Part model, mm, in its own coordinate system. Coordinates: 2 decimals unless noted, no trailing zeros. Loops run counter-clockwise (first coordinate to the right, second up) from the corner with the lowest first, then second, coordinate; pieces in that order, holes last. Notation, with made-up numbers: (34, -36) - (43, -36) arc R23 ccw to (43, -2) - close; hole circle Ø5 at (41.5, 83.25). An arc over 180 degrees is marked (long way). Use a Markdown table: item, result. Add a question column.
1) Band-saw the part on C-C (z = 10.5). Give the cut face in (x, y), plus the area to 3 significant figures.
2) Drop a flat-ended pin along its axis: P1, Ø3, axis at x = -77.4, z = 43.9, coming from the -Y side. Give the stop position or say it passes through.
3) Probe probe 1 along X at (y, z) = (2.9, -40); probe 2 along Z at (x, y) = (8, 3.5); probe 3 along X at (y, z) = (0.45, 41). List the from-to ranges inside material, lowest first. Write a range as [from, to].
4) Band-saw the part on D-D (y = 2.9). Give the number of separate pieces and of enclosed holes in the cut face, plus the area to 3 significant figures.
5) Band-saw the part on A-A (z = 40). Give the cut face in (x, y), plus the area to 3 significant figures.
6) Band-saw the part on B-B (x = -77.4). Give the cut face in (y, z).
from build123d import *

# Parameters (mm, degrees)
SKETCH1_W               = 161
SKETCH1_H               = 100
BOSS_EXTRUDE1_DEPTH     = 4
SKETCH2_R               = 1.75
CUT_EXTRUDE1_DEPTH      = 95.84856351
MIRROR2_COPY_1_SKETCH_R = 1.75
MIRROR2_COPY_1_DEPTH    = 95.84856351
SKETCH3_W               = 15
SKETCH3_H               = 60
CUT_EXTRUDE2_DEPTH      = 95.84856351
SKETCH4_R               = 1.6
CUT_EXTRUDE3_DEPTH      = 95.84856351
MIRROR5_COPY_1_SKETCH_R = 1.6
MIRROR5_COPY_1_DEPTH    = 95.84856351
SKETCH5_R               = 2.1
CUT_EXTRUDE4_DEPTH      = 95.84856351
SKETCH6_W               = 10
SKETCH6_H               = 40
CUT_EXTRUDE5_DEPTH      = 95.84856351
FILLET1_R               = 5


with BuildPart() as part:
    # Sketch1 → Boss-Extrude1 (new body)
    with BuildSketch(Plane(origin=(0, 0, 0), x_dir=(1, 0, 0), z_dir=(0, 1, 0))):
        Rectangle(SKETCH1_W, SKETCH1_H)
    extrude(amount=BOSS_EXTRUDE1_DEPTH)

    # Sketch2 → Cut-Extrude1 (cut, through all)
    with BuildSketch(Plane(origin=(0, 4, 0), x_dir=(1, 0, 0), z_dir=(0, 1, 0))):
        with Locations(Location((77.4, -43.9, 0), (0, 0, 270))):
            Circle(SKETCH2_R)
    cut_extrude1 = extrude(amount=-CUT_EXTRUDE1_DEPTH, mode=Mode.SUBTRACT)

    # Mirror1: Cut-Extrude1 across plane
    add(cut_extrude1.mirror(Plane.XY), mode=Mode.SUBTRACT)

    # Mirror2: Cut-Extrude1 across plane
    add(cut_extrude1.mirror(Plane(origin=(0, 0, 0), x_dir=(0, 0, 1), z_dir=(1, 0, 0))), mode=Mode.SUBTRACT)

    # Mirror2 copy 1 sketch → Mirror2 copy 1 (cut, through all)
    with BuildSketch(Plane(origin=(0, 4, 0), x_dir=(-1, 0, 0), z_dir=(0, 1, 0))):
        with Locations(Location((77.4, -43.9, 0), (0, 0, 270))):
            Circle(MIRROR2_COPY_1_SKETCH_R)
    extrude(amount=-MIRROR2_COPY_1_DEPTH, mode=Mode.SUBTRACT)

    # Sketch3 → Cut-Extrude2 (cut, through all)
    with BuildSketch(Plane(origin=(0, 4, 0), x_dir=(1, 0, 0), z_dir=(0, 1, 0))):
        with Locations((-27.5, -20)):
            Rectangle(SKETCH3_W, SKETCH3_H)
    cut_extrude2 = extrude(amount=-CUT_EXTRUDE2_DEPTH, mode=Mode.SUBTRACT)

    # Mirror3: Cut-Extrude2 across plane
    add(cut_extrude2.mirror(Plane(origin=(0, 0, 0), x_dir=(0, 0, 1), z_dir=(1, 0, 0))), mode=Mode.SUBTRACT)

    # Sketch4 → Cut-Extrude3 (cut, through all)
    with BuildSketch(Plane(origin=(0, 4, 0), x_dir=(1, 0, 0), z_dir=(0, 1, 0))):
        with Locations(Location((-70.5, 40, 0), (0, 0, 270))):
            Circle(SKETCH4_R)
    cut_extrude3 = extrude(amount=-CUT_EXTRUDE3_DEPTH, mode=Mode.SUBTRACT)

    # Mirror4: Cut-Extrude3 across plane
    add(cut_extrude3.mirror(Plane.XY), mode=Mode.SUBTRACT)

    # Mirror5: Cut-Extrude3 across plane
    add(cut_extrude3.mirror(Plane(origin=(0, 0, 0), x_dir=(0, 0, 1), z_dir=(1, 0, 0))), mode=Mode.SUBTRACT)

    # Mirror5 copy 1 sketch → Mirror5 copy 1 (cut, through all)
    with BuildSketch(Plane(origin=(0, 4, 0), x_dir=(-1, 0, 0), z_dir=(0, 1, 0))):
        with Locations(Location((-70.5, 40, 0), (0, 0, 270))):
            Circle(MIRROR5_COPY_1_SKETCH_R)
    extrude(amount=-MIRROR5_COPY_1_DEPTH, mode=Mode.SUBTRACT)

    # Sketch5 → Cut-Extrude4 (cut, through all)
    with BuildSketch(Plane(origin=(0, 4, 0), x_dir=(1, 0, 0), z_dir=(0, 1, 0))):
        with Locations(Location((-7.5, 10, 0), (0, 0, 270))):
            Circle(SKETCH5_R)
        with Locations(Location((7.5, 10, 0), (0, 0, 270))):
            Circle(SKETCH5_R)
        with Locations(Location((7.5, -10, 0), (0, 0, 270))):
            Circle(SKETCH5_R)
        with Locations(Location((-7.5, -10, 0), (0, 0, 270))):
            Circle(SKETCH5_R)
    extrude(amount=-CUT_EXTRUDE4_DEPTH, mode=Mode.SUBTRACT)

    # Sketch6 → Cut-Extrude5 (cut, through all)
    with BuildSketch(Plane(origin=(0, 4, 0), x_dir=(1, 0, 0), z_dir=(0, 1, 0))):
        with Locations((-65.5, 0)):
            Rectangle(SKETCH6_W, SKETCH6_H)
    cut_extrude5 = extrude(amount=-CUT_EXTRUDE5_DEPTH, mode=Mode.SUBTRACT)

    # Mirror6: Cut-Extrude5 across plane
    add(cut_extrude5.mirror(Plane(origin=(0, 0, 0), x_dir=(0, 0, 1), z_dir=(1, 0, 0))), mode=Mode.SUBTRACT)

    # Fillet1
    fillet1_edges = [part.edges().sort_by_distance(p)[0] for p in [
        (-20, 2, -10),
        (-35, 2, -10),
        (20, 2, -10),
        (35, 2, -10),
        (20, 2, 50),
        (35, 2, 50),
        (-20, 2, 50),
        (-35, 2, 50),
        (-80.5, 2, 50),
        (-80.5, 2, -50),
        (80.5, 2, -50),
        (80.5, 2, 50),
        (60.5, 2, -20),
        (70.5, 2, -20),
        (70.5, 2, 20),
        (60.5, 2, 20),
        (-70.5, 2, -20),
        (-60.5, 2, -20),
        (-60.5, 2, 20),
        (-70.5, 2, 20),
    ]]
    fillet(fillet1_edges, radius=FILLET1_R - 0.0001)  # a hair under: the kernel refuses the full size


solid = part.part
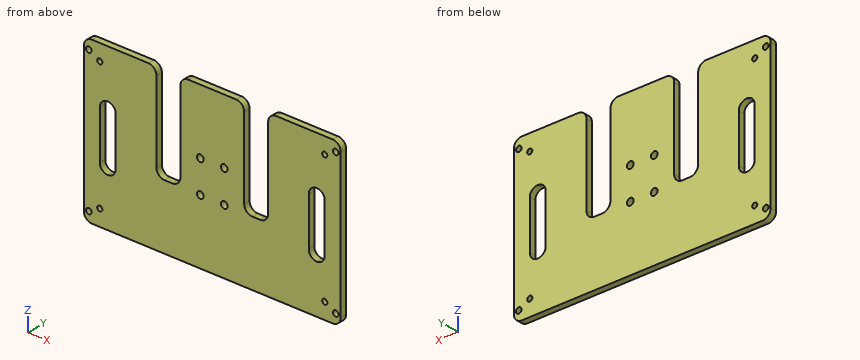
Answer block:
| question | item | result |
|---|---|---|
| 1 | outline | (-80.5, 0) - (-70.5, 0) - (-70.5, 4) - (-80.5, 4) - close; (-60.5, 0) - (-35, 0) - (-35, 4) - (-60.5, 4) - close; (-20, 0) - (-9.54, 0) - (-9.54, 4) - (-20, 4) - close; (-5.46, 0) - (5.46, 0) - (5.46, 4) - (-5.46, 4) - close; (9.54, 0) - (20, 0) - (20, 4) - (9.54, 4) - close; (35, 0) - (60.5, 0) - (60.5, 4) - (35, 4) - close; (70.5, 0) - (80.5, 0) - (80.5, 4) - (70.5, 4) - close |
| 1 | area | 411 mm2 |
| 2 | P1 | through |
| 3 | probe 1 | [-80.5, -72.1], [-68.9, 68.9], [72.1, 80.5] |
| 3 | probe 2 | [-50, -12.04], [-7.96, 7.96], [12.04, 50] |
| 3 | probe 3 | [-80.5, -71.75], [-69.25, -35], [-20, 20], [35, 69.25], [71.75, 80.5] |
| 4 | separate pieces | 1 |
| 4 | enclosed holes | 14 |
| 4 | area | 13,400 mm2 |
| 5 | outline | (-80.5, 0) - (-72.1, 0) - (-72.1, 4) - (-80.5, 4) - close; (-68.9, 0) - (-35, 0) - (-35, 4) - (-68.9, 4) - close; (-20, 0) - (20, 0) - (20, 4) - (-20, 4) - close; (35, 0) - (68.9, 0) - (68.9, 4) - (35, 4) - close; (72.1, 0) - (80.5, 0) - (80.5, 4) - (72.1, 4) - close |
| 5 | area | 498 mm2 |
| 6 | outline | (0, -49.62) - (4, -49.62) - (4, -45.65) - (0, -45.65) - close; (0, -42.15) - (4, -42.15) - (4, 42.15) - (0, 42.15) - close; (0, 45.65) - (4, 45.65) - (4, 49.62) - (0, 49.62) - close |
